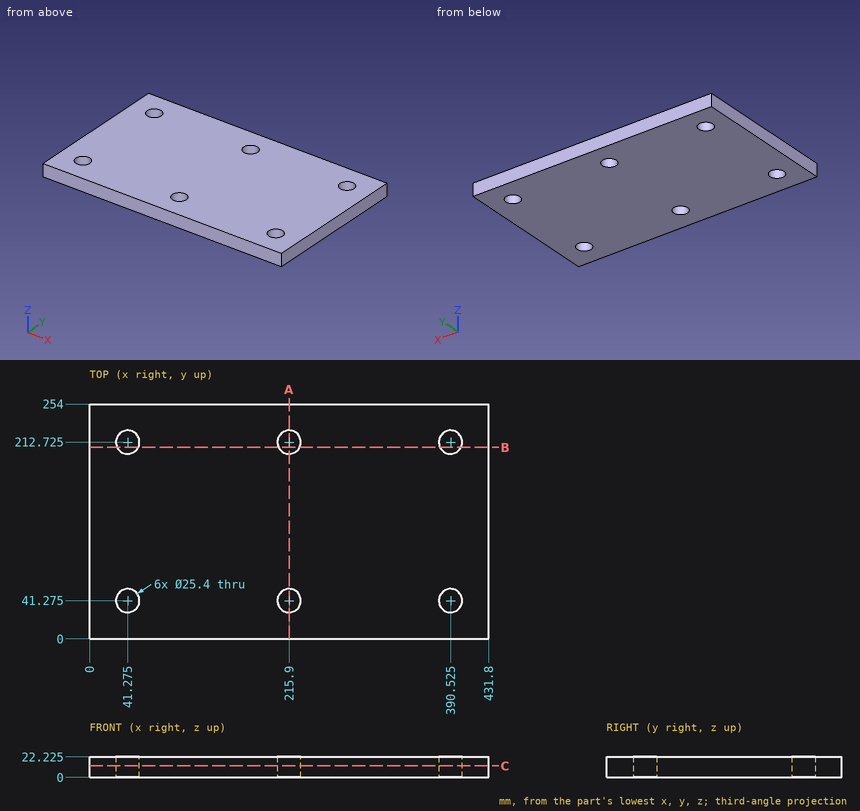
Design review of the part shown in the three views and the two pictorial views. Dimensions are in mm from the part's minimum x, y and z. Round coordinates to 2 decimals unless told otherwise and drop trailing zeros. Loops run counter-clockwise (first coordinate to the right, second up) from the corner with the lowest first, then second, coordinate; pieces in that order, holes last. Notation, with made-up numbers: (8.5, -4.5) -> (36.5, -4.5) arc R34 cw to (36.5, 32.5) -> close; hole circle Ø2 at (41, 25). An arc over 180 degrees is marked (long way). Answer as CSV lines item,"result".
1) To check wall thickness, follow line 1 along X through (y, z) = (30.5, 5.5). State the ranges of the line that lie inside material, in increasing order. Write a range as from..to.
Geometry results:
line 1,"x = 0..34.55, 48..209.18, 222.62..383.8, 397.25..431.8"
2) Add section C-C on z = 12.5. Write out the cut boundary in (x, y) (3 decimals), plus the area to 3 significant figures.
Geometry results:
outline,"(0, 0) -> (431.8, 0) -> (431.8, 254) -> (0, 254) -> close; hole circle Ø25.4 at (41.275, 41.275); hole circle Ø25.4 at (41.275, 212.725); hole circle Ø25.4 at (215.9, 41.275); hole circle Ø25.4 at (215.9, 212.725); hole circle Ø25.4 at (390.525, 41.275); hole circle Ø25.4 at (390.525, 212.725)"
area,"107,000 mm²"
3) Add section A-A on x = 215.9. Write out the cut boundary in (y, z) (3 decimals), plus the area to 3 significant figures.
Geometry results:
outline,"(0, 0) -> (28.575, 0) -> (28.575, 22.225) -> (0, 22.225) -> close; (53.975, 0) -> (200.025, 0) -> (200.025, 22.225) -> (53.975, 22.225) -> close; (225.425, 0) -> (254, 0) -> (254, 22.225) -> (225.425, 22.225) -> close"
area,"4,520 mm²"
4) Add section B-B on y = 207. Write out the cut boundary in (x, z) (3 decimals), plus the area to 3 significant figures.
Geometry results:
outline,"(0, 0) -> (29.939, 0) -> (29.939, 22.225) -> (0, 22.225) -> close; (52.611, 0) -> (204.564, 0) -> (204.564, 22.225) -> (52.611, 22.225) -> close; (227.236, 0) -> (379.189, 0) -> (379.189, 22.225) -> (227.236, 22.225) -> close; (401.861, 0) -> (431.8, 0) -> (431.8, 22.225) -> (401.861, 22.225) -> close"
area,"8,090 mm²"
